from build123d import *

# Parameters (mm, degrees)
BOSS_EXTRUDE1_START     = 12.827
BOSS_EXTRUDE1_DEPTH     = 6.35
F_1_4_CLEARANCE_HOLE1_D = 6.7564
FILLET1_R               = 6.35


with BuildPart() as part:
    # Sketch1 → Boss-Extrude1 (new body)
    with BuildSketch(Plane(origin=(0, 144.904574554, 0), x_dir=(-1, 0, 0), z_dir=(0, -1, 0)).offset(BOSS_EXTRUDE1_START)):
        with BuildLine():
            Line((-105.441812484, -1122.100334154), (-105.441812484, -1137.975334154))
            ThreePointArc((-105.441812484, -1137.975334154), (-114.966812484, -1147.500334154), (-124.491812484, -1137.975334154))
            Line((-124.491812484, -1137.975334154), (-124.491812484, -1087.175334154))
            ThreePointArc((-124.491812484, -1087.175334154), (-114.966812484, -1077.650334154), (-105.441812484, -1087.175334154))
            Line((-105.441812484, -1087.175334154), (-105.441812484, -1103.050334154))
            Line((-105.441812484, -1103.050334154), (-64.166812484, -1103.050334154))
            ThreePointArc((-64.166812484, -1103.050334154), (-54.641812484, -1112.575334154), (-64.166812484, -1122.100334154))
            Line((-64.166812484, -1122.100334154), (-105.441812484, -1122.100334154))
        make_face()
    extrude(amount=BOSS_EXTRUDE1_DEPTH)

    # 1/4 Clearance Hole1 (through all)
    with Locations(Plane(origin=(0, 125.727574554, 0), x_dir=(-1, 0, 0), z_dir=(0, -1, 0))):
        with Locations((-114.966812484, -1137.975334154), (-114.966812484, -1112.369211098), (-114.966812484, -1087.128841033), (-64.166812484, -1112.575334154), (-89.566812484, -1112.575334154)):
            Hole(F_1_4_CLEARANCE_HOLE1_D / 2)


with BuildPart() as body_2:
    # Mirror1: mirrored copy
    add(part.part.mirror(Plane(origin=(0, 0, 0), x_dir=(0, 0, 1), z_dir=(1, 0, 0))))

    # Fillet1
    fillet1_edges = [body_2.edges().sort_by_distance(p)[0] for p in [
        (-105.441812484, 128.902574554, 1122.100334154),
        (-105.441812484, 128.902574554, 1103.050334154),
    ]]
    fillet(fillet1_edges, radius=FILLET1_R)


solid = body_2.part
Verification items for the finished model (mm, model axes). A direction names the side the tool comes from. Give positions to 0.01 mm unless a question says otherwise; leave off trailing zeros. Loops run counter-clockwise (first coordinate to the right, second up) from the corner with the lowest first, then second, coordinate; pieces in that order, holes last.
1) Sectioned sample at C-C, the plane y = 131. Enter the section's corners in (x, z) (3 decimals), then the cut area to 3 significant figures.
2) Thickness scan on line 1 along Z through (x, y) = (-89.5, 127.75); line 2 along X through (y, z) = (130.25, 1113); line 3 along X through (y, z) = (131.25, 1138.5). Record the ranges inside material, lowest first.
3) Sectioned sample at B-B, the plane x = -91. Enter the section's corners in (y, z), then the cut area to 3 significant figures.
4) Sectioned sample at D-D, the plane x = -74.5. Enter the section's corners in (y, z), then the cut area to 3 significant figures.
5) Draft check along Z on faces 1 (the flat face through (-81, 129, 1122.1)), 2 (the flat face through (-82, 129, 1103.05)), 3 (the cylindrical face through (-114.527, 128.947, 1134.626)). Enter one of: pulls with the +Z half, pulls with the -Z half, needs draft (parallel to the pull), parting line crosses it, or undercut.
6) Set-up check for faces 4 (the flat face through (-105.442, 129, 1092)), 5 (the cylindrical face through (-116.526, 128.947, 1090.126)), 6 (the flat face through (-105.442, 129, 1133)): record each of +Z, -Z, +X, -X, +Y, -Y from which the full face is reachable in a straight line by a thin tool's end or side.
7) Depth check by flat-ended pin: pin 1 Ø2 at (x, y) = (-64.5, 130.5) entering from -Z; pin 2 Ø11 at (x, z) = (-114.97, 1137.98) entering from +Y; pin 3 Ø3 at (y, z) = (129, 1093) entering from +X; pin 4 Ø1.5 at (x, y) = (-111, 127) entering from -Z. Enter the tip coordinate at first touch or a pass-through.
8) Sectioned sample at A-A, the plane z = 1088.5. Enter the section's corners in (x, y), then the cut area to 3 significant figures.
Answers:
1. outline: (-124.492, 1087.175) arc R9.525 ccw to (-105.442, 1087.175) - (-105.442, 1096.7) arc R6.35 cw to (-99.092, 1103.05) - (-64.167, 1103.05) arc R9.525 ccw to (-64.167, 1122.1) - (-99.092, 1122.1) arc R6.35 cw to (-105.442, 1128.45) - (-105.442, 1137.975) arc R9.525 ccw to (-124.492, 1137.975) - close; hole circle Ø6.756 at (-114.967, 1087.129); hole circle Ø6.756 at (-114.967, 1112.369); hole circle Ø6.756 at (-114.967, 1137.975); hole circle Ø6.756 at (-89.567, 1112.575); hole circle Ø6.756 at (-64.167, 1112.575)
1. area: 2,020 mm2
2. line 1: z = 1103.05 to 1109.2, 1115.95 to 1122.1
2. line 2: x = -124.49 to -118.29, -111.65 to -92.92, -86.22 to -67.52, -60.82 to -54.65
2. line 3: x = -124.48 to -118.3, -111.63 to -105.46
3. outline: (125.73, 1103.05) - (132.08, 1103.05) - (132.08, 1109.52) - (125.73, 1109.52) - close; (125.73, 1115.63) - (132.08, 1115.63) - (132.08, 1122.1) - (125.73, 1122.1) - close
3. area: 82.1 mm2
4. outline: (125.73, 1103.05) - (132.08, 1103.05) - (132.08, 1122.1) - (125.73, 1122.1) - close
4. area: 121 mm2
5. face 1: pulls with the +Z half
5. face 2: pulls with the -Z half
5. face 3: undercut
6. face 4: -Z, +X, +Y, -Y
6. face 5: +Y, -Y
6. face 6: +Z, +X, +Y, -Y
7. pin 1: stops at z = 1103.05
7. pin 2: stops at y = 132.08
7. pin 3: stops at x = -105.44
7. pin 4: stops at z = 1078.21
8. outline: (-124.49, 125.73) - (-118.05, 125.73) - (-118.05, 132.08) - (-124.49, 132.08) - close; (-111.88, 125.73) - (-105.44, 125.73) - (-105.44, 132.08) - (-111.88, 132.08) - close
8. area: 81.8 mm2
